from build123d import *

# Parameters (mm, degrees)
CORTAR_EXTRUIR1_DEPTH                          = 34
PERFORADOR_PARA_ROSCAR_PARA_MACHO_DE_ROS_D     = 4.2
PERFORADOR_PARA_ROSCAR_PARA_MACHO_DE_ROS_DEPTH = 40
PERFORADOR_PARA_ROSCAR_PARA_MACHO_DE_ROS_TIP   = 1.2618073
PERFORADOR_PARA_ROSCAR_PARA_MACHO_DE_2_D       = 4.2
PERFORADOR_PARA_ROSCAR_PARA_MACHO_DE_2_DEPTH   = 40
PERFORADOR_PARA_ROSCAR_PARA_MACHO_DE_2_TIP     = 1.2618073


with BuildPart() as part:
    # Croquis1 → Revolución1 (revolve)
    with BuildSketch(Plane.XY, mode=Mode.PRIVATE) as revoluci_n1_sk:
        Polygon((0, 0), (34, 0), (34, 38), (20, 38), (20, 101.6), (16.35, 101.6), (11.767282238, 93.6625), (8.232717762, 93.6625), (3.65, 101.6), (0, 101.6), align=None)
    revolve(revoluci_n1_sk.sketch.rotate(Axis((0, 0, 0), (1, 0, 0)), 90), axis=Axis((0, 0, 0), (1, 0, 0)))

    # Croquis2 → Cortar-Extruir1 (cut)
    with BuildSketch(Plane(origin=(34, 0, 0), x_dir=(0, 0, -1), z_dir=(1, 0, 0))):
        with BuildLine():
            Line((-3, 9.5), (3, 9.5))
            Line((3, 9.5), (3, 6.873863542))
            ThreePointArc((3, 6.873863542), (0, -7.5), (-3, 6.873863542))
            Line((-3, 6.873863542), (-3, 9.5))
        make_face()
    extrude(amount=-CORTAR_EXTRUIR1_DEPTH, mode=Mode.SUBTRACT)

    # Perforador para roscar para macho de roscar para M51
    with Locations(Plane(origin=(27, 0, 38), x_dir=(1, 0, 0), z_dir=(0, 0, 1))):
        with Locations((0, 0)):
            Hole(PERFORADOR_PARA_ROSCAR_PARA_MACHO_DE_ROS_D / 2, depth=PERFORADOR_PARA_ROSCAR_PARA_MACHO_DE_ROS_DEPTH)
            with Locations((0, 0, -(PERFORADOR_PARA_ROSCAR_PARA_MACHO_DE_ROS_DEPTH + PERFORADOR_PARA_ROSCAR_PARA_MACHO_DE_ROS_TIP / 2))):  # 118° drill point
                Cone(0, PERFORADOR_PARA_ROSCAR_PARA_MACHO_DE_ROS_D / 2, PERFORADOR_PARA_ROSCAR_PARA_MACHO_DE_ROS_TIP, mode=Mode.SUBTRACT)

    # Perforador para roscar para macho de 2
    with Locations(Plane(origin=(27, 38, 0), x_dir=(0, 0, 1), z_dir=(0, 1, 0))):
        with Locations((0, 0)):
            Hole(PERFORADOR_PARA_ROSCAR_PARA_MACHO_DE_2_D / 2, depth=PERFORADOR_PARA_ROSCAR_PARA_MACHO_DE_2_DEPTH)
            with Locations((0, 0, -(PERFORADOR_PARA_ROSCAR_PARA_MACHO_DE_2_DEPTH + PERFORADOR_PARA_ROSCAR_PARA_MACHO_DE_2_TIP / 2))):  # 118° drill point
                Cone(0, PERFORADOR_PARA_ROSCAR_PARA_MACHO_DE_2_D / 2, PERFORADOR_PARA_ROSCAR_PARA_MACHO_DE_2_TIP, mode=Mode.SUBTRACT)


solid = part.part
Work out the finished part from the listing and answer in its coordinate system (mm). A direction names the side the tool comes from. Coordinates: 2 decimals unless noted, no trailing zeros. Use one line per item in the form item = value. Start each with the question number.
1. The mould has two halves that part along X. Classify faces 4 (the face through (7.946, -28.283, 89.811)), 5 (the face through (34, -1, -8)), 6 (the face through (17, 9.5, 0)), 7 (the face through (11.99, 57.23, -74.63)): released by +X, released by -X, zero draft, split by the parting line, or undercut.
2. Each of these flat-tipped pins is pushed along its axis until it touches: P1, Ø3.5, axis at x = 27, y = 0, coming from the -Z side; P2, Ø12, axis at y = 51, z = 30.5, coming from the +X side; P3, Ø12, axis at x = 4, z = 60, coming from the -Y side; P4, Ø9, axis at y = 0, z = 0, coming from the +X side. Where does it stop, or does it pass through?
3. Straight lines are drawn through the part: probe 1 along X at (y, z) = (0, 16); probe 2 along Y at (x, z) = (11, 0); probe 3 along X at (y, z) = (46.5, 68.5). For each, find the intervals that lie inside material, in ascending order. Write a range as from..to.
4. A tool of negligible diameter and unlimited length cuts with its end or side. For faces 1 (the face through (20, -1, -44)), 2 (the face through (17.238, -7.495, -0.287)), 3 (the face through (9.975, 91.435, -20.304)), from which of +Z, -Z, +X, -X, +Y, -Y can it reach the whole face along a straight path? Write none if from no direction.
Evaluation:
q1.face_4 = undercut
q1.face_5 = released by +X
q1.face_6 = zero draft
q1.face_7 = undercut
q2.P1 = -38
q2.P2 = 20
q2.P3 = -86.05
q2.P4 = through
q3.probe_1 = 0..24.9, 29.1..34
q3.probe_2 = -93.66..-7.5, 9.5..93.66
q3.probe_3 = 0..20
q4.face_1 = +X
q4.face_2 = +X, -X
q4.face_3 = none
